Input: part model. Units: mm. Frame: model coordinates. A direction names the side the tool comes from. Give positions to 0.01 mm unless a question says otherwise; leave off trailing zeros. Loops run counter-clockwise (first coordinate to the right, second up) from the corner with the lowest first, then second, coordinate; pieces in that order, holes last. Notation, with made-up numbers: M 89.5,37 L 133.5,37 A19 ccw 133.5,73 Z; hole C 13,40.5 d2. An arc over 180 degrees is marked long. Use CSV: the item, a comma, the result in double quotes. Start each with the question number.
Autodesk Inventor part; units mm, degrees
ref_plane "Plano de trabajo1" through (25.1, 0, 0) normal (1, 0, 0) x (0, 0, -1)
ref_plane "YZ Plane" through (0, 0, 0) normal (1, 0, 0) x (0, 1, 0)
ref_plane "XZ Plane" through (0, 0, 0) normal (0, 1, 0) x (-1, 0, 0)
sketch "Boceto1" plane through (0, 0, 0) normal (0, 1, 0) x (-1, 0, 0)
  line L0 (0, 0) -> (-50.2, 0)
  line L1 (-50.2, 0) -> (-50.2, -65.2)
  line L2 (-50.2, -65.2) -> (0, -65.2)
  line L3 (0, -65.2) -> (0, 0)
  dimension "d0" = 50.2
  dimension "d1" = 65.2
extrude "Extrusión1" add sketch "Boceto1" along normal blind 20.7
sketch "Boceto2" plane through (0, 20.7, 0) normal (0, 1, 0) x (1, 0, 0)
  line L0 (-14.4985, 32.6) -> (58.2485, 32.6)
  circle A0 centre (25.1, 32.6) radius 18.5
  line L1 (0, 65.2) -> (0, 0)
  dimension "d7" = 37
  dimension "d57" = 0
  dimension "d58" = 25.1
extrude "Extrusión2" cut sketch "Boceto2" against normal blind 15
sketch "Boceto3" plane through (50.2, 0, 0) normal (1, 0, 0) x (0, 0, -1)
  line L0 (32.6, 28.8672) -> (32.6, -9.3744)
  line L1 (-5.2256, 10.35) -> (70.0589, 10.35)
  line L2 (25.95, 10.35) -> (39.25, 10.35) construction
  line L3 (25.95, 8.85) -> (39.25, 8.85)
  line L4 (39.25, 11.85) -> (25.95, 11.85)
  arc A0 (25.95, 11.85) -> (25.95, 8.85) centre (25.95, 10.35) ccw
  arc A1 (39.25, 8.85) -> (39.25, 11.85) centre (39.25, 10.35) ccw
  point P0 (0, 0)
  point P1 (32.6, 10.35)
  point P2 (40.75, 10.35)
  point P3 (24.45, 10.35)
  dimension "d11" = 16.3
  dimension "d12" = 3
  dimension "d13" = 0
extrude "Extrusión3" cut sketch "Boceto3" against normal blind 4
chamfer "Chaflán1" distance 4 angle 45 4 edges at (50.2, 8.85, -32.6) (50.2, 10.35, -24.45) (50.2, 11.85, -32.6) (50.2, 10.35, -40.75)
sketch "Boceto4" plane through (50.2, 0, 0) normal (1, 0, 0) x (0, 0, -1)
  point P0 (0, 0)
ref_plane "Plano de trabajo1" through (25.1, 0, 0) normal (1, 0, 0) x (0, 0, -1)
mirror "Simetría1" about plane through (25.1, 0, 0) normal (1, 0, 0) of "Extrusión3"
chamfer "Chaflán2" distance 4 angle 45 4 edges at (0, 11.85, -32.6) (0, 10.35, -24.45) (0, 8.85, -32.6) (0, 10.35, -40.75)
chamfer "Chaflán3" distance 2.5 angle 45 1 edges at (6.6, 20.7, -32.6)
sketch "Boceto5" plane through (0, 0, 0) normal (0, -1, 0) x (1, 0, 0)
  line L0 (25.1, 22.2035) -> (25.1, -86.3829)
  line L1 (-10.0483, -32.6) -> (59.9656, -32.6)
  circle A0 centre (6.05, -7.2) radius 3.2
  circle A1 centre (44.15, -7.2) radius 3.2
  circle A2 centre (6.05, -58) radius 3.2
  circle A3 centre (31.45, -45.3) radius 3.2
  point P0 (0, 0)
  dimension "d35" = 38.1
  dimension "d36" = 38.1
  dimension "d37" = 0
  dimension "d38" = 50.8
  dimension "d39" = 50.8
  dimension "d40" = 12.7
  dimension "d41" = 12.7
  dimension "d42" = 6.4
extrude "Extrusión4" add sketch "Boceto5" along normal blind 4.2
fillet "Empalme1" radius 3.2 4 edges at (2.85, -4.2, -58) (28.25, -4.2, -45.3) (40.95, -4.2, -7.2) (2.85, -4.2, -7.2)
sketch "Boceto6" plane through (0, 20.7, 0) normal (0, 1, 0) x (1, 0, 0)
  line L0 (-6.6573, 32.6) -> (60.5927, 32.6)
  line L1 (25.1, -18.2708) -> (25.1, 82.1469)
  circle A0 centre (6.05, 13.55) radius 3.7
  circle A1 centre (6.05, 51.65) radius 3.7
  circle A2 centre (44.15, 13.55) radius 3.7
  circle A3 centre (44.15, 51.65) radius 3.7
  point P0 (0, 0)
  dimension "d51" = 38.1
  dimension "d52" = 38.1
  dimension "d53" = 38.1
  dimension "d54" = 38.1
  dimension "d55" = 38.1
  dimension "d56" = 7.4
extrude "Extrusión5" cut sketch "Boceto6" against normal blind 5
properties material "Plastico PETG"
Item 1: Set-up query: faces 4 (the flat face through (4, 10, -33)), 5 (the cylindrical face through (40.454, 18.235, -13.713)), 6 (the flat face through (46.2, 10, -32)). Return all of +Z, -Z, +X, -X, +Y, -Y with unobstructed straight access to the full face (end or side cutting, diameter ignored); none if empty.
Item 2: Material intervals for line 1 (Z direction, x = 44.15, y = 17.95); line 2 (Z direction, x = 25.1, y = 13); line 3 (X direction, y = 17.3, z = -13.55), sorted ascending.
Item 3: Section C-C (z = -58). Output: boundary loops of the cut face in (x, y), then the cut area to 3 significant figures.
Item 4: First-contact query: pin 1 Ø4 at (x, z) = (29.5, -42) entering from -Y; pin 2 Ø15 at (x, z) = (21, -33.5) entering from -Y; pin 3 Ø0.9 at (y, z) = (10, -32) entering from +X. Flat tips, straight axial feed; report the tip coordinate or a pass-through.
Item 5: Section B-B (x = 25.1). Output: boundary loops of the cut face in (y, z).
Item 6: Mould query, pull axis Z, two halves, no side actions, for faces 1 (the cylindrical face through (47.202, -0.493, -8.161)), 2 (the flat face through (25, 10, 0)), 3 (the conical face through (47.78, 10.42, -22.87)). Classes: +Z half, -Z half, draft (parallel to the pull), parting line (faces both ways), or undercut.
Recorded:
1,face 4,"-X"
1,face 5,"+Y"
1,face 6,"+X"
2,line 1,"-65.2 to -55.35, -47.95 to -17.25, -9.85 to 0"
2,line 2,"-65.2 to -51.1, -14.1 to 0"
2,line 3,"0 to 2.35, 9.75 to 40.45, 47.85 to 50.2"
3,outline,"M 0,0 L 2.85,0 L 2.85,-1 A3.2 ccw 9.25,-1 L 9.25,0 L 50.2,0 L 50.2,20.7 L 0,20.7 Z"
3,area,"1,060 mm²"
4,pin 1,"y = -3.62"
4,pin 2,"y = 0"
4,pin 3,"x = 46.2"
5,outline,"M 0,-65.2 L 20.7,-65.2 L 20.7,-53.6 L 18.2,-51.1 L 5.7,-51.1 L 5.7,-14.1 L 18.2,-14.1 L 20.7,-11.6 L 20.7,0 L 0,0 Z"
6,face 1,"parting line"
6,face 2,"+Z half"
6,face 3,"undercut"
